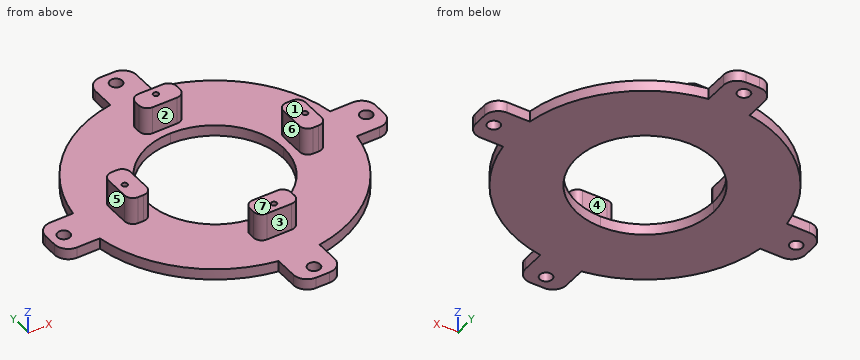
```python
from build123d import *

# Parameters (mm, degrees)
F1_DEPTH = 4
F0_W     = 7.5
F0_H     = 8
F0_W_2   = 8
F0_H_2   = 7.5
F2_DEPTH = 14
F4_D     = 2
F4_DEPTH = 11
F4_TIP   = 0.600860619
F5_D     = 4.5
F5_DEPTH = 11
F5_TIP   = 1.3519363928
F6_R     = 5
F7_R     = 3


with BuildPart() as f1:
    # F0 (on Top) → F1 (new body)
    with BuildSketch(Plane.XY):
        with BuildLine():
            Line((28, 0), (25, 0))
            ThreePointArc((25, 0), (17.6776695297, -17.6776695297), (0, -25))
            Line((0, -25), (0, -28))
            Line((0, -28), (7.5, -28))
            Line((7.5, -28), (7.5, -36))
            Line((7.5, -36), (7.5, -47.0307412763))
            ThreePointArc((7.5, -47.0307412763), (33.675960454, -33.675960454), (47.0307412763, -7.5))
            Line((47.0307412763, -7.5), (36, -7.5))
            Line((36, -7.5), (28, -7.5))
            Line((28, -7.5), (28, 0))
        make_face()
        with BuildLine():
            ThreePointArc((0, 25), (17.6776695297, 17.6776695297), (25, 0))
            Line((25, 0), (28, 0))
            Line((28, 0), (28, 7.5))
            Line((28, 7.5), (36, 7.5))
            Line((36, 7.5), (47.0307412763, 7.5))
            ThreePointArc((47.0307412763, 7.5), (33.675960454, 33.675960454), (7.5, 47.0307412763))
            Line((7.5, 47.0307412763), (7.5, 36))
            Line((7.5, 36), (7.5, 28))
            Line((7.5, 28), (0, 28))
            Line((0, 28), (0, 25))
        make_face()
        with BuildLine():
            ThreePointArc((-25, 0), (-17.6776695297, 17.6776695297), (0, 25))
            Line((0, 25), (0, 28))
            Line((0, 28), (-7.5, 28))
            Line((-7.5, 28), (-7.5, 36))
            Line((-7.5, 36), (-7.5, 47.0307412763))
            ThreePointArc((-7.5, 47.0307412763), (-33.675960454, 33.675960454), (-47.0307412763, 7.5))
            Line((-47.0307412763, 7.5), (-36, 7.5))
            Line((-36, 7.5), (-28, 7.5))
            Line((-28, 7.5), (-28, 0))
            Line((-28, 0), (-25, 0))
        make_face()
        with BuildLine():
            Line((0, -28), (0, -25))
            ThreePointArc((0, -25), (-17.6776695297, -17.6776695297), (-25, 0))
            Line((-25, 0), (-28, 0))
            Line((-28, 0), (-28, -7.5))
            Line((-28, -7.5), (-36, -7.5))
            Line((-36, -7.5), (-47.0307412763, -7.5))
            ThreePointArc((-47.0307412763, -7.5), (-33.675960454, -33.675960454), (-7.5, -47.0307412763))
            Line((-7.5, -47.0307412763), (-7.5, -36))
            Line((-7.5, -36), (-7.5, -28))
            Line((-7.5, -28), (0, -28))
        make_face()
        with BuildLine():
            Line((36, 7.5), (36, 0))
            Line((36, 0), (47.625, 0))
            ThreePointArc((47.625, 0), (47.476202872, 3.7617530299), (47.0307412763, 7.5))
            Line((47.0307412763, 7.5), (36, 7.5))
        make_face()
        with BuildLine():
            Line((47.625, 0), (36, 0))
            Line((36, 0), (36, -7.5))
            Line((36, -7.5), (47.0307412763, -7.5))
            ThreePointArc((47.0307412763, -7.5), (47.476202872, -3.7617530299), (47.625, 0))
        make_face()
        with BuildLine():
            Line((-7.5, 36), (0, 36))
            Line((0, 36), (0, 47.625))
            ThreePointArc((0, 47.625), (-3.7617530299, 47.476202872), (-7.5, 47.0307412763))
            Line((-7.5, 47.0307412763), (-7.5, 36))
        make_face()
        with BuildLine():
            Line((0, 47.625), (0, 36))
            Line((0, 36), (7.5, 36))
            Line((7.5, 36), (7.5, 47.0307412763))
            ThreePointArc((7.5, 47.0307412763), (3.7617530299, 47.476202872), (0, 47.625))
        make_face()
        with BuildLine():
            Line((7.5, -36), (0, -36))
            Line((0, -36), (0, -47.625))
            ThreePointArc((0, -47.625), (3.7617530299, -47.476202872), (7.5, -47.0307412763))
            Line((7.5, -47.0307412763), (7.5, -36))
        make_face()
        with BuildLine():
            Line((0, -47.625), (0, -36))
            Line((0, -36), (-7.5, -36))
            Line((-7.5, -36), (-7.5, -47.0307412763))
            ThreePointArc((-7.5, -47.0307412763), (-3.7617530299, -47.476202872), (0, -47.625))
        make_face()
        with BuildLine():
            ThreePointArc((47.0307412763, 7.5), (47.476202872, 3.7617530299), (47.625, 0))
            ThreePointArc((47.625, 0), (47.476202872, -3.7617530299), (47.0307412763, -7.5))
            Line((47.0307412763, -7.5), (60.325, -7.5))
            Line((60.325, -7.5), (60.325, 7.5))
            Line((60.325, 7.5), (47.0307412763, 7.5))
        make_face()
        with BuildLine():
            Line((-36, -7.5), (-36, 0))
            Line((-36, 0), (-47.625, 0))
            ThreePointArc((-47.625, 0), (-47.476202872, -3.7617530299), (-47.0307412763, -7.5))
            Line((-47.0307412763, -7.5), (-36, -7.5))
        make_face()
        with BuildLine():
            Line((-47.625, 0), (-36, 0))
            Line((-36, 0), (-36, 7.5))
            Line((-36, 7.5), (-47.0307412763, 7.5))
            ThreePointArc((-47.0307412763, 7.5), (-47.476202872, 3.7617530299), (-47.625, 0))
        make_face()
        with BuildLine():
            ThreePointArc((-7.5, 47.0307412763), (-3.7617530299, 47.476202872), (0, 47.625))
            ThreePointArc((0, 47.625), (3.7617530299, 47.476202872), (7.5, 47.0307412763))
            Line((7.5, 47.0307412763), (7.5, 60.325))
            Line((7.5, 60.325), (-7.5, 60.325))
            Line((-7.5, 60.325), (-7.5, 47.0307412763))
        make_face()
        with BuildLine():
            ThreePointArc((7.5, -47.0307412763), (3.7617530299, -47.476202872), (0, -47.625))
            ThreePointArc((0, -47.625), (-3.7617530299, -47.476202872), (-7.5, -47.0307412763))
            Line((-7.5, -47.0307412763), (-7.5, -60.325))
            Line((-7.5, -60.325), (7.5, -60.325))
            Line((7.5, -60.325), (7.5, -47.0307412763))
        make_face()
        with BuildLine():
            ThreePointArc((-47.0307412763, -7.5), (-47.476202872, -3.7617530299), (-47.625, 0))
            ThreePointArc((-47.625, 0), (-47.476202872, 3.7617530299), (-47.0307412763, 7.5))
            Line((-47.0307412763, 7.5), (-60.325, 7.5))
            Line((-60.325, 7.5), (-60.325, -7.5))
            Line((-60.325, -7.5), (-47.0307412763, -7.5))
        make_face()
    extrude(amount=F1_DEPTH)

    # F0 (on Top) → F2 (join)
    with BuildSketch(Plane.XY):
        with Locations((3.75, 32)):
            Rectangle(F0_W, F0_H)
        with Locations((-3.75, 32)):
            Rectangle(F0_W, F0_H)
        with Locations((32, 3.75)):
            Rectangle(F0_W_2, F0_H_2)
        with Locations((32, -3.75)):
            Rectangle(F0_W_2, F0_H_2)
        with Locations((3.75, -32)):
            Rectangle(F0_W, F0_H)
        with Locations((-3.75, -32)):
            Rectangle(F0_W, F0_H)
        with Locations((-32, -3.75)):
            Rectangle(F0_W_2, F0_H_2)
        with Locations((-32, 3.75)):
            Rectangle(F0_W_2, F0_H_2)
    extrude(amount=F2_DEPTH)

    # F4
    with Locations(Plane.XY.offset(14)):
        with Locations((0, 33), (33, 0), (0, -33), (-33, 0)):
            Hole(F4_D / 2, depth=F4_DEPTH)
            with Locations((0, 0, -(F4_DEPTH + F4_TIP / 2))):  # 118° drill point
                Cone(0, F4_D / 2, F4_TIP, mode=Mode.SUBTRACT)

    # F5
    with Locations(Plane(origin=(0, 0, 0), x_dir=(1, 0, 0), z_dir=(0, 0, -1))):
        with Locations((0, -55.325), (55.325, 0), (0, 55.325), (-55.325, 0)):
            Hole(F5_D / 2, depth=F5_DEPTH)
            with Locations((0, 0, -(F5_DEPTH + F5_TIP / 2))):  # 118° drill point
                Cone(0, F5_D / 2, F5_TIP, mode=Mode.SUBTRACT)

    # F6
    f6_edges = [f1.edges().sort_by_distance(p)[0] for p in [
        (7.5, 60.325, 2),
        (-7.5, 60.325, 2),
        (-60.325, 7.5, 2),
        (-60.325, -7.5, 2),
        (7.5, -60.325, 2),
        (-7.5, -60.325, 2),
        (60.325, -7.5, 2),
        (60.325, 7.5, 2),
    ]]
    fillet(f6_edges, radius=F6_R)

    # F7
    f7_edges = [f1.edges().sort_by_distance(p)[0] for p in [
        (7.5, 28, 9),
        (7.5, 36, 9),
        (-7.5, 28, 9),
        (-7.5, 36, 9),
        (-36, -7.5, 9),
        (-28, -7.5, 9),
        (-36, 7.5, 9),
        (-28, 7.5, 9),
        (-7.5, -28, 9),
        (7.5, -28, 9),
        (36, 7.5, 9),
        (28, 7.5, 9),
        (36, -7.5, 9),
        (28, -7.5, 9),
        (7.5, -36, 9),
        (-7.5, -36, 9),
    ]]
    fillet(f7_edges, radius=F7_R)


solid = f1.part
```
Model file for the job. Use its own axes, mm. Face numbers are marked on the shaded views. A direction names the side the tool comes from. Give positions to 0.01 mm unless a question says otherwise; leave off trailing zeros. Loops run counter-clockwise (first coordinate to the right, second up) from the corner with the lowest first, then second, coordinate; pieces in that order, holes last. Notation, with made-up numbers: (6.25, -35) -> (62.25, -35) arc R11 ccw to (62.25, -14) -> close; hole circle Ø9 at (-11.5, 53). An arc over 180 degrees is marked (long way). Write each question's results on one line, items separated by ' | '.
(1) Cut at D-D on x = 49.5. List the corners of the cut face in (y, z), and give its area (3 significant figures).
Geometry results:
outline: (-7.5, 0) -> (7.5, 0) -> (7.5, 4) -> (-7.5, 4) -> close | area: 60.0 mm²
(2) Flat gauge pins, fed straight in: pin 1 Ø1.2 at (y, z) = (53, 1.5) entering from -X; pin 2 Ø0.6 at (y, z) = (-32, 9.5) entering from +X; pin 3 Ø12 at (x, y) = (-0.5, -21) entering from +Z; pin 4 Ø2 at (x, y) = (30, 24.5) entering from -Z. Where does each tip first touch, or does it go through?
Geometry results:
pin 1: stops at x = -7.5 | pin 2: stops at x = 7.5 | pin 3: stops at z = 4 | pin 4: stops at z = 0
(3) Cut at B-B on y = -15.5. List the corners of the cut face in (x, z).
Geometry results:
outline: (-45.03, 0) -> (-19.62, 0) -> (-19.62, 4) -> (-45.03, 4) -> close; (19.62, 0) -> (45.03, 0) -> (45.03, 4) -> (19.62, 4) -> close
(4) Pull direction Y, two halves, no side cores. Call the marked faces 1, 2 and 3: released by +Y, released by -Y, zero draft, split by the parting line, or undercut.
Geometry results:
face 1: zero draft | face 2: undercut | face 3: released by -Y
(5) Probe line 1 along Y through (x, z) = (0, 12.25); line 2 along X through (y, z) = (4.5, 11); line 3 along Y through (x, z) = (33, 6.75). List the from-to ranges inside material, lowest first.
Geometry results:
line 1: y = -36 to -34, -32 to -28, 28 to 32, 34 to 36 | line 2: x = -36 to -28, 28 to 36 | line 3: y = -7.5 to -1, 1 to 7.5
(6) Tool access for the marked faces 4, 5, 6 and 7: list every direction of +Z, -Z, +X, -X, +Y, -Y with a clear straight run to the whole face (end or side of a thin tool).
Geometry results:
face 4: +Z, +X, -X | face 5: +Z, -X, +Y, -Y | face 6: +Z, +Y, -Y | face 7: +Z, +X, -X, +Y, -Y
(7) Cut at A-A on x = 23. List the corners of the cut face in (y, z), and give its area (3 significant figures).
Geometry results:
outline: (-41.7, 0) -> (-9.8, 0) -> (-9.8, 4) -> (-41.7, 4) -> close; (9.8, 0) -> (41.7, 0) -> (41.7, 4) -> (9.8, 4) -> close | area: 255 mm²
(8) Cut at C-C on z = 10. Give the number of separate pieces and of enclosed holes in the cut face, and give its area (3 significant figures).
Geometry results:
separate pieces: 4 | enclosed holes: 4 | area: 437 mm²
